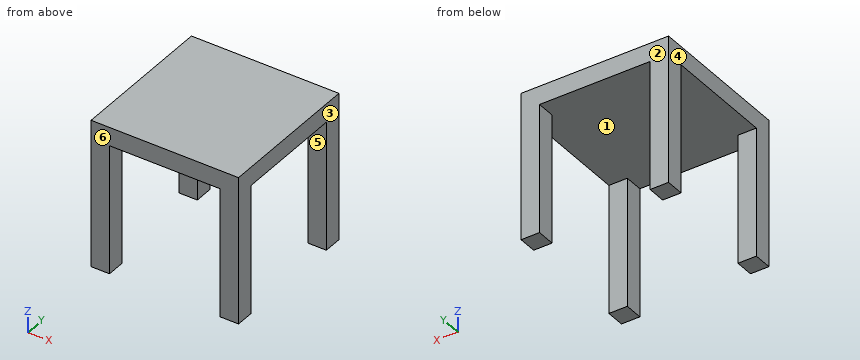
from build123d import *

# Parameters (mm, degrees)
F1_W     = 800
F1_H     = 800
F2_DEPTH = 100
F0_W     = 100
F0_H     = 100
F3_DEPTH = 700


with BuildPart() as f2:
    # F1 (on Top) → F2 (new body)
    with BuildSketch(Plane.XY):
        with Locations((400, 400)):
            Rectangle(F1_W, F1_H)
    extrude(amount=F2_DEPTH)

    # F0 (on Top) → F3 (join)
    with BuildSketch(Plane.XY):
        with Locations((50, 50)):
            Rectangle(F0_W, F0_H)
        with Locations((750, 50)):
            Rectangle(F0_W, F0_H)
        with Locations((50, 750)):
            Rectangle(F0_W, F0_H)
        with Locations((750, 750)):
            Rectangle(F0_W, F0_H)
    extrude(amount=-F3_DEPTH)


solid = f2.part
CAD build for the part. Positions are in the model's coordinates, mm. Face numbers are marked on the shaded views. A direction names the side the tool comes from. Coordinates: 2 decimals unless noted, no trailing zeros. Order: outer loops, then holes, each group sorted by start corner. A loop starts at its lowest first (then second) coordinate and runs counter-clockwise, first axis right, second up. Notation, with made-up numbers: (-35.5, 68.5) -> (-23.5, 68.5) arc R18 cw to (-23.5, 87.5) -> close; hole circle Ø4 at (57, 59). An arc over 180 degrees is marked (long way). Answer in a Markdown table with one row per item.
1) Which spindle directions (+Z, -Z, +X, -X, +Y, -Y) get a long thin tool onto all of the face, cutting with end or side? Do the marked faces 5 and 6. Say none if no direction does.
Check values:
| item | result |
|---|---|
| face 5 | -Z, +X, -X |
| face 6 | +Z, -Z, +X, -X, -Y |
2) Band-saw the part on B-B (y = 70.5). List the corners of the cut face in (x, z).
Check values:
| item | result |
|---|---|
| outline | (0, -700) -> (100, -700) -> (100, 0) -> (700, 0) -> (700, -700) -> (800, -700) -> (800, 100) -> (0, 100) -> close |
3) Mould opens along X. For the marked faces 1, 2, 3 and 4 say: pulls with the +X half, pulls with the -X half, needs draft (parallel to the pull), parting line crosses it, or undercut.
Check values:
| item | result |
|---|---|
| face 1 | undercut |
| face 2 | needs draft |
| face 3 | pulls with the +X half |
| face 4 | pulls with the -X half |
4) Band-saw the part on D-D (y = 570). List the corners of the cut face in (x, z), and give its area (3 significant figures).
Check values:
| item | result |
|---|---|
| outline | (0, 0) -> (800, 0) -> (800, 100) -> (0, 100) -> close |
| area | 80,000 mm2 |
5) Band-saw the part on A-A (z = -497.5). List the corners of the cut face in (x, y), and give its area (3 significant figures).
Check values:
| item | result |
|---|---|
| outline | (0, 0) -> (100, 0) -> (100, 100) -> (0, 100) -> close; (0, 700) -> (100, 700) -> (100, 800) -> (0, 800) -> close; (700, 0) -> (800, 0) -> (800, 100) -> (700, 100) -> close; (700, 700) -> (800, 700) -> (800, 800) -> (700, 800) -> close |
| area | 40,000 mm2 |
6) Flat gauge pin, fed straight in: P1, Ø4, axis at x = 440, y = 118.5, coming from the -Z side. Where does the tip first touch, or does it go through?
Check values:
| item | result |
|---|---|
| P1 | z = 0 |
7) Drill centre lines: line 1 (X direction, y = 76.5, z = -478); line 2 (Z direction, x = 160.5, y = 709.5). Where is each one in solid material? Low to high.
Check values:
| item | result |
|---|---|
| line 1 | 0 to 100, 700 to 800 |
| line 2 | 0 to 100 |
